Read the model definition and answer for the solid it produces. Units are mm, in the model's axes. Coordinates: 2 decimals unless noted, no trailing zeros. Loops run counter-clockwise (first coordinate to the right, second up) from the corner with the lowest first, then second, coordinate; pieces in that order, holes last.
from build123d import *

# Parameters (mm, degrees)
SKETCH1_W           = 81.3
SKETCH1_H           = 50.8
SKETCH1_R           = 1.5
BOSS_EXTRUDE1_DEPTH = 1.6
CHAMFER1_SIZE       = 1


with BuildPart() as part:
    # Sketch1 → Boss-Extrude1 (new body)
    with BuildSketch(Plane.XY):
        with Locations((40.65, 25.4)):
            Rectangle(SKETCH1_W, SKETCH1_H)
        with Locations((5.1, 25.4)):
            Circle(SKETCH1_R, mode=Mode.SUBTRACT)
        with Locations((40.65, 25.4)):
            Circle(SKETCH1_R, mode=Mode.SUBTRACT)
        with Locations((76.2, 25.4)):
            Circle(SKETCH1_R, mode=Mode.SUBTRACT)
    extrude(amount=BOSS_EXTRUDE1_DEPTH)

    # Chamfer1
    chamfer1_edges = [part.edges().sort_by_distance(p)[0] for p in [
        (0, 50.8, 0.8),
        (81.3, 50.8, 0.8),
        (81.3, 0, 0.8),
        (0, 0, 0.8),
    ]]
    chamfer(chamfer1_edges, length=CHAMFER1_SIZE)


solid = part.part
Q1. Determine the mould class of faces 1 (the face through (42.036, 24.825, 0.789)), 2 (the face through (0, 25, 1)), 3 (the face through (40, 50.8, 1)) for opening direction Y: +Y half, -Y half, draft (parallel to the pull), parting line (faces both ways), or undercut.
Findings below:
face 1: undercut
face 2: draft
face 3: +Y half
Q2. A cutting plane is placed at C-C (x = 41). Give the vertices of the cut face in (y, z), then the cut area to 3 significant figures.
Findings below:
outline: (0, 0) - (23.94, 0) - (23.94, 1.6) - (0, 1.6) - close; (26.86, 0) - (50.8, 0) - (50.8, 1.6) - (26.86, 1.6) - close
area: 76.6 mm2
Q3. A cutting plane is placed at A-A (x = 5.1). Give the vertices of the cut face in (y, z), then the cut area to 3 significant figures.
Findings below:
outline: (0, 0) - (23.9, 0) - (23.9, 1.6) - (0, 1.6) - close; (26.9, 0) - (50.8, 0) - (50.8, 1.6) - (26.9, 1.6) - close
area: 76.5 mm2
Q4. A cutting plane is placed at B-B (y = 25.4). Give the vertices of the cut face in (x, z).
Findings below:
outline: (0, 0) - (3.6, 0) - (3.6, 1.6) - (0, 1.6) - close; (6.6, 0) - (39.15, 0) - (39.15, 1.6) - (6.6, 1.6) - close; (42.15, 0) - (74.7, 0) - (74.7, 1.6) - (42.15, 1.6) - close; (77.7, 0) - (81.3, 0) - (81.3, 1.6) - (77.7, 1.6) - close
Q5. A flat-ended cylindrical pin translates along its axis: pin 1 Ø1.8 at (x, y) = (76.2, 25.4) entering from +Z. Find the tip coordinate at first contact, or state that the pin passes through.
Findings below:
pin 1: passes through
Q6. A straight line is drawn through the part: probe 1 along Y at (x, z) = (40.65, 0.4). Find the intervals that lie inside material, in ascending order.
Findings below:
probe 1: y = 0 to 23.9, 26.9 to 50.8
